Read the model definition and answer for the solid it produces. Units are mm, in the model's axes. Face numbers are marked on the shaded views. A direction names the side the tool comes from. Coordinates: 2 decimals unless noted, no trailing zeros. Order: outer loops, then holes, each group sorted by start corner. A loop starts at its lowest first (then second) coordinate and runs counter-clockwise, first axis right, second up. Notation, with made-up numbers: M 57,-4.5 L 65,-4.5 A15 cw 65,13.5 Z; hole C -38,13 d9. An arc over 180 degrees is marked long. Use a Markdown table: item, result. Add a question column.
1) Find section C-C on y = -23.5. Write down the section's boundary in (x, z), plus the area to 3 significant figures.
2) Find section D-D on x = -11. Write down the section's boundary in (y, z), plus the area to 3 significant figures.
3) The mould has two halves that part along Z. Classify the marked faces 5, 6, 7 and 8: released by +Z, released by -Z, zero draft, split by the parting line, or undercut.
4) Find section A-A on z = 0. Write down the section's boundary in (x, y), plus the area to 3 significant figures.
5) For the marked faces 1, 2, 3 and 4, determine the directions among +Z, -Z, +X, -X, +Y, -Y from which every point of the face is accessible in a straight line to the end or side of a thin tool.
6) Each of these flat-tipped pins is pushed along its axis until it touches: pin 1 Ø5.5 at (x, z) = (54, 0.5) entering from +Y; pin 2 Ø7.5 at (y, z) = (-5, 2) entering from +X; pin 3 Ø7.5 at (y, z) = (-2, 0.5) entering from -X. Where does it stop, or does it pass through?
7) Find the intervals of material crossed by probe 1 along X at (y, z) = (-43.75, 0); probe 2 along X at (y, z) = (-38, 0); probe 3 along Z at (x, y) = (50, -47.5), in increasing order. Write a range as [from, to].
8) Find section B-B on x = -50. Write down the section's boundary in (y, z), plus the area to 3 significant figures.
Autodesk Inventor part; units mm, degrees
ref_plane "YZ Plane" through (0, 0, 0) normal (1, 0, 0) x (0, 1, 0)
ref_plane "XZ Plane" through (0, 0, 0) normal (0, 1, 0) x (-1, 0, 0)
ref_plane "XY Plane" through (0, 0, 0) normal (0, 0, 1) x (1, 0, 0)
sketch "Sketch1" plane through (0, 0, 0) normal (0, 0, 1) x (1, 0, 0)
  line L0 (-60, 0) -> (60, 0)
  line L1 (60, 0) -> (60, -52)
  line L2 (60, -52) -> (-60, -52)
  line L3 (-60, -52) -> (-60, 0)
  line L4 (0, -62.4) -> (0, 10.4)
  point P0 (0, 0)
  dimension "d0" = 120
  dimension "d1" = 52
extrude "Extrusion1" add sketch "Sketch1" along normal mid plane 80
sketch "Sketch2" plane through (-60, 0, 40) normal (0, 1, 0) x (1, 0, 0)
  line L0 (47.5, 49.5) -> (72.5, 49.5)
  line L1 (72.5, 49.5) -> (72.5, 30.5)
  line L2 (72.5, 30.5) -> (47.5, 30.5)
  line L3 (47.5, 30.5) -> (47.5, 49.5)
  line L4 (-24, 40) -> (144, 40)
  line L5 (60, 96) -> (60, -16)
  point P0 (60, 40)
  dimension "d4" = 19
  dimension "d5" = 25
extrude "Extrusion2" cut sketch "Sketch2" against normal blind 7
sketch "Sketch3" plane through (-60, 0, 40) normal (0, 1, 0) x (1, 0, 0)
  point P0 (60, 40)
  point P1 (60, 40)
hole "Hole1" at (0, 0, 0) direction (0, -1, 0) diameter 12 end through all
sketch "Sketch4" plane through (-60, 0, 40) normal (0, 1, 0) x (1, 0, 0)
  line L0 (-24, 40) -> (144, 40)
  line L1 (60, 96) -> (60, -16)
  point P0 (60, 40)
  point P1 (10, 40)
  point P2 (110, 40)
  dimension "d15" = 50
hole "Hole2" at (-50, 0, 0) at (50, 0, 0) direction (0, -1, 0) diameter 5 end through all
sketch "Sketch5" plane through (0, 0, 0) normal (0, 0, 1) x (1, 0, 0)
  circle A0 centre (0, 43) radius 10.1
  line L0 (0, 43) -> (42, 35.5943)
  line L1 (60, 0) -> (-60, 0)
  line L2 (42, 35.5943) -> (42, 0)
  line L3 (22, 0) -> (22, 39.1208)
  line L4 (22, 0) -> (42, 0)
  line L5 (0, -10.62) -> (0, 63.72)
  line L6 (0, 43) -> (-42, 35.5943)
  line L7 (-60, 0) -> (60, 0)
  line L8 (-42, 35.5943) -> (-42, 0)
  line L9 (-22, 0) -> (-22, 39.1208)
  point P0 (0, 0)
  dimension "d23" = 22
  dimension "d24" = 42
  dimension "d29" = 10
extrude "Extrusion3" add sketch "Sketch5" along normal mid plane 80 contours L0 L2 L1 L3 | L9 L1 L8 L6
sketch "Sketch6" plane through (42, 0, 40) normal (1, 0, 0) x (0, 0, -1)
  line L0 (20, 0) -> (60, 0)
  line L1 (60, 0) -> (60, 44.1208)
  line L2 (60, 44.1208) -> (20, 44.1208)
  line L3 (20, 44.1208) -> (20, 0)
  line L4 (80, 35.5943) -> (80, 0)
  line L5 (0, 0) -> (0, 35.5943)
  line L6 (80, 39.1208) -> (0, 39.1208)
  point P0 (40, 0)
  dimension "d30" = 20
  dimension "d31" = 20
  dimension "d32" = 5
extrude "Extrusion4" cut sketch "Sketch6" against normal through all
sketch "Sketch7" plane through (-60, 0, 40) normal (0, 1, 0) x (1, 0, 0)
  line L0 (0, 0) -> (0, 80)
  line L1 (18, 20) -> (18, 0)
  line L2 (0, 80) -> (18, 80)
  line L3 (18, 80) -> (18, 0)
  line L4 (18, 0) -> (0, 0)
  line L5 (0, 0) -> (0, 80)
  line L6 (120, 0) -> (102, 0)
  line L7 (102, 80) -> (102, 60)
  line L8 (120, 0) -> (102, 0)
  line L9 (102, 0) -> (102, 80)
  line L10 (102, 80) -> (120, 80)
  line L11 (120, 80) -> (120, 0)
  point P0 (60, 40)
extrude "Extrusion5" cut sketch "Sketch7" against normal blind 40
fillet "Fillet1" radius 20 2 edges at (-42, 0, 0) (42, 0, 0)
equation "\"d31\" = d30"
properties part number "Foot_Ankl_Connector"
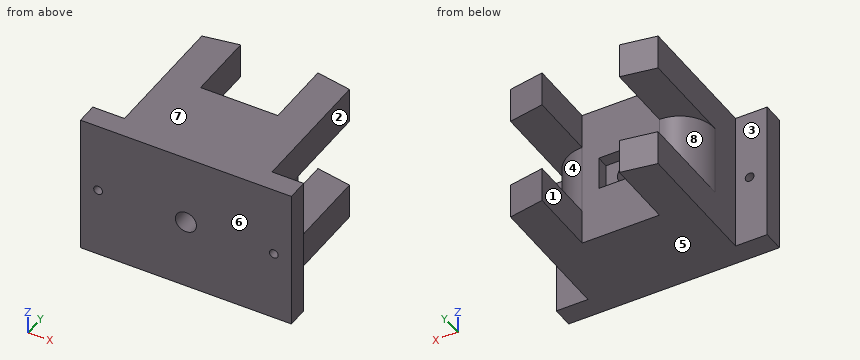
Check result:
| question | item | result |
|---|---|---|
| 1 | outline | M -42,-40 L 42,-40 L 42,40 L -42,40 Z; hole C 0,0 d12 |
| 1 | area | 6,610 mm2 |
| 2 | outline | M -52,-40 L 0,-40 L 0,-9.5 L -7,-9.5 L -7,9.5 L 0,9.5 L 0,40 L -52,40 Z |
| 2 | area | 4,030 mm2 |
| 3 | face 5 | released by -Z |
| 3 | face 6 | zero draft |
| 3 | face 7 | released by +Z |
| 3 | face 8 | undercut |
| 4 | outline | M -60,-52 L -52.5,-52 L -52.5,-40 L -60,-40 Z; M -47.5,-52 L -6,-52 L -6,-7 L -12.5,-7 L -12.5,0 L -22,0 A20 ccw -42,-20 L -42,-40 L -47.5,-40 Z; M 6,-52 L 47.5,-52 L 47.5,-40 L 42,-40 L 42,-20 A20 ccw 22,0 L 12.5,0 L 12.5,-7 L 6,-7 Z; M 52.5,-52 L 60,-52 L 60,-40 L 52.5,-40 Z |
| 4 | area | 3,790 mm2 |
| 5 | face 1 | +Z, -Z, +Y |
| 5 | face 2 | +Z, -Z, +X, +Y |
| 5 | face 3 | +Z, -Z, -X, +Y |
| 5 | face 4 | +X, +Y |
| 6 | pin 1 | stops at y = -40 |
| 6 | pin 2 | stops at x = 38.54 |
| 6 | pin 3 | stops at x = -36.03 |
| 7 | probe 1 | x = [-60, -52.5], [-47.5, -6], [6, 47.5], [52.5, 60] |
| 7 | probe 2 | x = [-42, -6], [6, 42] |
| 7 | probe 3 | z = [-40, -2.5], [2.5, 40] |
| 8 | outline | M -52,-40 L -40,-40 L -40,-2.5 L -52,-2.5 Z; M -52,2.5 L -40,2.5 L -40,40 L -52,40 Z |
| 8 | area | 900 mm2 |
